```python
from build123d import *

# Parameters (mm, degrees)
BOSS_EXTRUDE1_DEPTH = 6.35
SKETCH2_W           = 6.35
SKETCH2_H           = 12.7
BOSS_EXTRUDE2_DEPTH = 6.35
FILLET1_R           = 2.54
FILLET2_R           = 1.27
SKETCH3_R           = 2
CUT_EXTRUDE1_DEPTH  = 6.35


with BuildPart() as part:
    # Sketch1 → Boss-Extrude1 (new body)
    with BuildSketch(Plane.XY):
        with BuildLine():
            Line((0, 0), (0, 7.62))
            ThreePointArc((0, 7.62), (1.487897552, 11.212102448), (5.08, 12.7))
            Line((5.08, 12.7), (12.7, 12.7))
            Line((12.7, 12.7), (12.7, 6.35))
            Line((12.7, 6.35), (114.3, 6.35))
            Line((114.3, 6.35), (114.3, 12.7))
            Line((114.3, 12.7), (115.57, 12.7))
            ThreePointArc((115.57, 12.7), (119.162102448, 11.212102448), (120.65, 7.62))
            Line((120.65, 7.62), (120.65, 4.57332967))
            ThreePointArc((120.65, 4.57332967), (119.34544285, 1.174442898), (116.101798705, -0.478758031))
            Line((116.101798705, -0.478758031), (5.611798705, -12.109284347))
            ThreePointArc((5.611798705, -12.109284347), (1.681113228, -10.832639496), (0, -7.057196646))
            Line((0, -7.057196646), (0, 0))
        make_face()
    extrude(amount=BOSS_EXTRUDE1_DEPTH)

    # Sketch2 → Boss-Extrude2 (add)
    with BuildSketch(Plane(origin=(0, 0, 0), x_dir=(-1, 0, 0), z_dir=(0, 0, -1))):
        with Locations((-15.875, 0)):
            Rectangle(SKETCH2_W, SKETCH2_H)
    extrude(amount=BOSS_EXTRUDE2_DEPTH)

    # Fillet1
    fillet1_edges = [part.edges().sort_by_distance(p)[0] for p in [
        (19.05, 0, 0),
    ]]
    fillet(fillet1_edges, radius=FILLET1_R)

    # Fillet2
    fillet2_edges = [part.edges().sort_by_distance(p)[0] for p in [
        (67.945, 6.35, 0),
        (63.5, 6.35, 6.35),
        (19.05, 6.35, -4.445),
        (19.793948776, 6.35, -0.743948776),
    ]]
    fillet(fillet2_edges, radius=FILLET2_R)

    # Sketch3 → Cut-Extrude1 (cut)
    with BuildSketch(Plane(origin=(0, 0, 0), x_dir=(-1, 0, 0), z_dir=(0, 0, -1))):
        with Locations((-5.08, 7.62)):
            Circle(SKETCH3_R)
    extrude(amount=-CUT_EXTRUDE1_DEPTH, mode=Mode.SUBTRACT)


solid = part.part
```
The listing builds one solid part. Answer for the finished solid, in the listing's coordinates (mm). A direction names the side the tool comes from. Give positions to 0.01 mm unless a question says otherwise; leave off trailing zeros. Loops run counter-clockwise (first coordinate to the right, second up) from the corner with the lowest first, then second, coordinate; pieces in that order, holes last. Notation, with made-up numbers: M 6.25,76.5 L 58.25,76.5 A32 cw 58.25,112.5 Z; hole C 31,47.25 d1. An arc over 180 degrees is marked long. One line per item, written item: value.
Q1. Flat-ended cylindrical pins translate along their axes: P1, Ø12.5, axis at x = 41, y = 3.5, coming from the -Z side; P2, Ø1.9, axis at y = -3.5, z = -3.5, coming from the +X side; P3, Ø3, axis at y = 1, z = -2, coming from the -X side. Find the tip coordinate at first contact, or state that the pin passes through.
Working result:
P1: stops at z = 0
P2: stops at x = 19.05
P3: stops at x = 12.7
Q2. Determine the mould class of faces 1 (the face through (114.3, 10, 3)), 2 (the face through (12.7, 0, -3)), 3 (the face through (48, 0, 6.35)) for opening direction X: +X half, -X half, draft (parallel to the pull), parting line (faces both ways), or undercut.
Working result:
face 1: undercut
face 2: -X half
face 3: draft
Q3. A cutting plane is placed at C-C on x = 41. Determine the outline of the cut face in (y, z).
Working result:
outline: M -8.38,0 L 5.08,0 A1.27 ccw 6.35,1.27 L 6.35,5.08 A1.27 ccw 5.08,6.35 L -8.38,6.35 Z
Q4. A cutting plane is placed at B-B on x = 73.5. Determine the outline of the cut face in (y, z), then the cut area to 3 significant figures.
Working result:
outline: M -4.96,0 L 5.08,0 A1.27 ccw 6.35,1.27 L 6.35,5.08 A1.27 ccw 5.08,6.35 L -4.96,6.35 Z
area: 71.1 mm^2
Q5. A cutting plane is placed at A-A on y = -4. Determine the outline of the cut face in (x, z), then the cut area to 3 significant figures.
Working result:
outline: M 0,0 L 12.7,0 L 12.7,-6.35 L 19.05,-6.35 L 19.05,-2.54 A2.54 cw 21.59,0 L 82.65,0 L 82.65,6.35 L 0,6.35 Z
area: 567 mm^2
Q6. For faces 4 (the face through (3.233, 6.854, 3.131)), 5 (the face through (60, 6.35, 3)), 6 (the face through (16, -6.35, -3)), 7 (the face through (61.63, -6.213, 3.131)), 8 (the face through (19.05, -1, -4)), determine the directions among +Z, -Z, +X, -X, +Y, -Y from which every point of the face is accessible in a straight line to the end or side of a thin tool.
Working result:
face 4: +Z, -Z
face 5: +Z, -Z, +Y
face 6: -Z, +X, -X, -Y
face 7: +Z, -Z, +X, -Y
face 8: -Z, +X, +Y, -Y
Q7. Find the intervals of material crossed by line 1 (Y direction, x = 5.08, z = 3); line 2 (Z direction, x = 92.5, y = -0.75); line 3 (X direction, y = 3.25, z = -2.25), in increasing order. Write a range as from..to.
Working result:
line 1: y = -12.14..5.62, 9.62..12.7
line 2: z = 0..6.35
line 3: x = 12.7..19.07
